Read the model definition and answer for the solid it produces. Units are mm, in the model's axes. Face numbers are marked on the shaded views. Give positions to 0.01 mm unless a question says otherwise; leave off trailing zeros. Loops run counter-clockwise (first coordinate to the right, second up) from the corner with the lowest first, then second, coordinate; pieces in that order, holes last. Notation, with made-up numbers: (21.25, 55.25) - (41.25, 55.25) arc R34 ccw to (41.25, 86.25) - close; hole circle Ø8 at (57.25, 56.5). An arc over 180 degrees is marked (long way). Write each question's results on one line, items separated by ' | '. Start each with the question number.
Q1. The part is cut by section A-A, the plane x = 0. Write down the section's boundary in (y, z).
Q2. The part is cut by section C-C, the plane x = -12.25. Write down the section's boundary in (y, z).
Q3. The part is cut by section D-D, the plane y = 8.5. Write down the section's boundary in (x, z), plus the area to 3 significant figures.
Q4. Determine the mould class of the marked faces 1, 2, 3 and 4 for opening direction Y: +Y half, -Y half, draft (parallel to the pull), parting line (faces both ways), or undercut.
Q5. Given pin 1 (1.5 mm diameter, centred on x = 4, z = 1, fed in from -Y); pin 2 (2.5 mm diameter, centred on x = 12.56, y = -7.32, fed in from -Z); pin 3 (8 mm diameter, centred on x = 10.5, y = -5, fed in from +Z), each flat-ended and moving along its own axis, determine where each tip first touches the part or whether it passes through.
Q6. Find the intervals of material crossed by line 1 (X direction, y = -8, z = 1.8); line 2 (X direction, y = -7, z = 1.6); line 3 (Y direction, x = 1, z = 0.85), in increasing order. Write a range as from..to.
Q7. The part is cut by section B-B, the plane z = 2. Write down the section's boundary in (x, y), plus the area to 3 significant figures.
```python
from build123d import *

# Parameters (mm, degrees)
F0_R     = 1.5
F1_DEPTH = 3
F2_W     = 2.2
F2_H     = 2.2
F3_DEPTH = 0.2
F5_DEPTH = 0.1
F6_DEPTH = 0.2


with BuildPart() as f1:
    # F0 (on Top) → F1 (new body)
    with BuildSketch(Plane.XY):
        with BuildLine():
            ThreePointArc((5.053231, 11.711225), (3.778342, 12.753574), (3.24572, 14.311827))
            ThreePointArc((3.24572, 14.311827), (0, 17.395082), (-3.24572, 14.311827))
            ThreePointArc((-3.24572, 14.311827), (-3.778342, 12.753574), (-5.053231, 11.711225))
            ThreePointArc((-5.053231, 11.711225), (-11.046083, 6.377459), (-12.668834, -1.479386))
            ThreePointArc((-12.668834, -1.479386), (-12.93409, -3.104647), (-14.017265, -4.345038))
            ThreePointArc((-14.017265, -4.345038), (-15.14542, -8.548699), (-11.080733, -10.104918))
            ThreePointArc((-11.080733, -10.104918), (-9.449522, -9.788391), (-7.900064, -10.388572))
            ThreePointArc((-7.900064, -10.388572), (-0.067306, -13.051011), (7.792495, -10.469501))
            ThreePointArc((7.792495, -10.469501), (9.332641, -9.886588), (10.948438, -10.20445))
            ThreePointArc((10.948438, -10.20445), (15.444934, -8.940161), (14.180645, -4.443665))
            ThreePointArc((14.180645, -4.443665), (14.098171, -4.395651), (14.017265, -4.345038))
            ThreePointArc((14.017265, -4.345038), (12.93409, -3.104647), (12.668834, -1.479386))
            ThreePointArc((12.668834, -1.479386), (11.046083, 6.377459), (5.053231, 11.711225))
        make_face()
        with Locations((-12.25, -7.072541)):
            Circle(F0_R, mode=Mode.SUBTRACT)
        with Locations((12.564541, -7.324058)):
            Circle(F0_R, mode=Mode.SUBTRACT)
        with Locations((0, 14.145082)):
            Circle(F0_R, mode=Mode.SUBTRACT)
    extrude(amount=F1_DEPTH)

    # F2 (on face) → F3 (join)
    with BuildSketch(Plane.XY.offset(3)):
        with Locations((0, -0.504918)):
            Rectangle(F2_W, F2_H)
    extrude(amount=F3_DEPTH)

    # F4 (on face) → F5 (join)
    with BuildSketch(Plane.XY.offset(3)):
        with BuildLine():
            Line((-4.80058, -10.782232), (-3.42495, -8.286207))
            ThreePointArc((-3.42495, -8.286207), (-4.327749, -7.852521), (-5.176546, -7.320852))
            Line((-5.176546, -7.320852), (-6.552177, -9.816877))
            ThreePointArc((-6.552177, -9.816877), (-5.696863, -10.336723), (-4.80058, -10.782232))
        make_face()
        with BuildLine():
            Line((-2.94705, -11.428779), (-2.471803, -8.618683))
            ThreePointArc((-2.471803, -8.618683), (-2.953059, -8.465869), (-3.42495, -8.286207))
            Line((-3.42495, -8.286207), (-4.80058, -10.782232))
            ThreePointArc((-4.80058, -10.782232), (-3.88728, -11.144108), (-2.94705, -11.428779))
        make_face()
        with BuildLine():
            ThreePointArc((-0.499806, -8.952189), (-1.495132, -8.840593), (-2.471803, -8.618683))
            Line((-2.471803, -8.618683), (-2.94705, -11.428779))
            ThreePointArc((-2.94705, -11.428779), (-1.968128, -11.637378), (-0.975053, -11.762286))
            Line((-0.975053, -11.762286), (-0.499806, -8.952189))
        make_face()
        with BuildLine():
            ThreePointArc((0.499806, -8.952189), (0, -8.966131), (-0.499806, -8.952189))
            Line((-0.499806, -8.952189), (-0.975053, -11.762286))
            ThreePointArc((-0.975053, -11.762286), (0, -11.802631), (0.975053, -11.762286))
            Line((0.975053, -11.762286), (0.499806, -8.952189))
        make_face()
        with BuildLine():
            ThreePointArc((2.471803, -8.618683), (1.495132, -8.840593), (0.499806, -8.952189))
            Line((0.499806, -8.952189), (0.975053, -11.762286))
            ThreePointArc((0.975053, -11.762286), (1.968128, -11.637378), (2.94705, -11.428779))
            Line((2.94705, -11.428779), (2.471803, -8.618683))
        make_face()
        with BuildLine():
            ThreePointArc((3.42495, -8.286207), (2.953059, -8.465869), (2.471803, -8.618683))
            Line((2.471803, -8.618683), (2.94705, -11.428779))
            ThreePointArc((2.94705, -11.428779), (3.88728, -11.144108), (4.80058, -10.782232))
            Line((4.80058, -10.782232), (3.42495, -8.286207))
        make_face()
        with BuildLine():
            ThreePointArc((5.176546, -7.320852), (4.327749, -7.852521), (3.42495, -8.286207))
            Line((3.42495, -8.286207), (4.80058, -10.782232))
            ThreePointArc((4.80058, -10.782232), (5.696863, -10.336723), (6.552177, -9.816877))
            Line((6.552177, -9.816877), (5.176546, -7.320852))
        make_face()
    extrude(amount=F5_DEPTH)

    # F4 (on face) → F6 (join)
    with BuildSketch(Plane.XY.offset(3)):
        with BuildLine():
            Line((-4.80058, -10.782232), (-3.42495, -8.286207))
            ThreePointArc((-3.42495, -8.286207), (-4.327749, -7.852521), (-5.176546, -7.320852))
            Line((-5.176546, -7.320852), (-6.552177, -9.816877))
            ThreePointArc((-6.552177, -9.816877), (-5.696863, -10.336723), (-4.80058, -10.782232))
        make_face()
        with BuildLine():
            ThreePointArc((-0.499806, -8.952189), (-1.495132, -8.840593), (-2.471803, -8.618683))
            Line((-2.471803, -8.618683), (-2.94705, -11.428779))
            ThreePointArc((-2.94705, -11.428779), (-1.968128, -11.637378), (-0.975053, -11.762286))
            Line((-0.975053, -11.762286), (-0.499806, -8.952189))
        make_face()
        with BuildLine():
            ThreePointArc((2.471803, -8.618683), (1.495132, -8.840593), (0.499806, -8.952189))
            Line((0.499806, -8.952189), (0.975053, -11.762286))
            ThreePointArc((0.975053, -11.762286), (1.968128, -11.637378), (2.94705, -11.428779))
            Line((2.94705, -11.428779), (2.471803, -8.618683))
        make_face()
        with BuildLine():
            ThreePointArc((5.176546, -7.320852), (4.327749, -7.852521), (3.42495, -8.286207))
            Line((3.42495, -8.286207), (4.80058, -10.782232))
            ThreePointArc((4.80058, -10.782232), (5.696863, -10.336723), (6.552177, -9.816877))
            Line((6.552177, -9.816877), (5.176546, -7.320852))
        make_face()
    extrude(amount=F6_DEPTH)


solid = f1.part
```
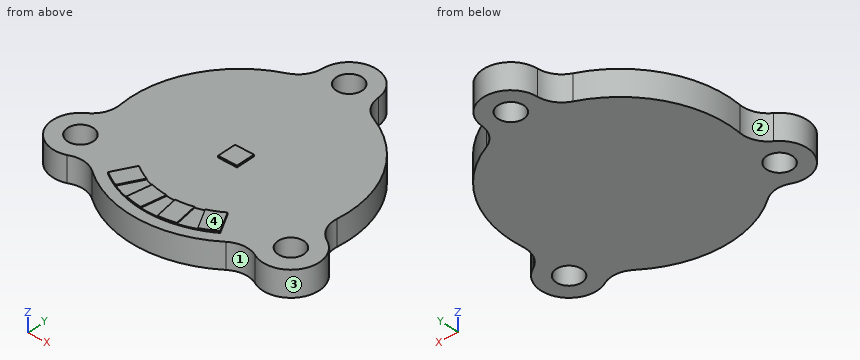
Check sheet entries:
1) outline: (-13.05, 0) - (12.65, 0) - (12.65, 3) - (0.6, 3) - (0.6, 3.2) - (-1.6, 3.2) - (-1.6, 3) - (-8.97, 3) - (-8.97, 3.1) - (-11.8, 3.1) - (-11.8, 3) - (-13.05, 3) - close; (15.65, 0) - (17.4, 0) - (17.4, 3) - (15.65, 3) - close
2) outline: (-10.32, 0) - (-8.57, 0) - (-8.57, 3) - (-10.32, 3) - close; (-5.57, 0) - (3.55, 0) - (3.55, 3) - (-5.57, 3) - close
3) outline: (-9.51, 0) - (9.51, 0) - (9.51, 3) - (-9.51, 3) - close | area: 57.1 mm^2
4) face 1: -Y half | face 2: undercut | face 3: parting line | face 4: draft
5) pin 1: stops at y = -12.64 | pin 2: passes through | pin 3: stops at z = 3
6) line 1: x = -15.36..-13.43, -11.07..11.23, 13.9..15.8 | line 2: x = -15.5..-13.75, -10.75..11.1, 14.03..15.85 | line 3: y = -13.01..13.03, 15.26..17.24
7) outline: (-14.02, -4.35) arc R3.25 ccw to (-11.08, -10.1) arc R3 cw to (-7.9, -10.39) arc R13.05 ccw to (7.79, -10.47) arc R3 cw to (10.95, -10.2) arc R3.3 ccw to (14.18, -4.44) arc R3 cw to (14.02, -4.35) arc R3 cw to (12.67, -1.48) arc R12.75 ccw to (5.05, 11.71) arc R3 cw to (3.25, 14.31) arc R3.25 ccw to (-3.25, 14.31) arc R3 cw to (-5.05, 11.71) arc R12.75 ccw to (-12.67, -1.48) arc R3 cw to start; hole circle Ø3 at (-12.25, -7.07); hole circle Ø3 at (0, 14.15); hole circle Ø3 at (12.56, -7.32) | area: 583 mm^2
